The model under review builds one solid part; all positions refer to its coordinate system, in mm. A direction names the side the tool comes from. Give positions to 0.01 mm unless a question says otherwise; leave off trailing zeros. Loops run counter-clockwise (first coordinate to the right, second up) from the corner with the lowest first, then second, coordinate; pieces in that order, holes last. Notation, with made-up numbers: (22, -13) - (50, -13) arc R20 ccw to (50, 10) - close; hole circle Ø7 at (-34, -38). An arc over 180 degrees is marked (long way). Return JSON: item names as keys, results as strings. Group by question number.
from build123d import *

# Parameters (mm, degrees)
SKETCH1_W             = 60
SKETCH1_H             = 50
BOSS_EXTRUDE1_DEPTH   = 3
SKETCH2_W             = 10
SKETCH2_H             = 3
CUT_EXTRUDE1_DEPTH    = 3
CAVITY3_START         = -30
CAVITY3_OUTLINE_W     = 7
CAVITY3_OUTLINE_H     = 3
CAVITY3_OUTLINE_W_2   = 10
CAVITY3_DEPTH         = 3
CAVITY3_START_2       = 27
CAVITY3_2_OUTLINE_W   = 7
CAVITY3_2_OUTLINE_H   = 3
CAVITY3_2_OUTLINE_W_2 = 10
CAVITY3_2_DEPTH       = 3


# Read off the part's stored shape, not the designer's step: Cavity3
with BuildPart() as part:
    # Sketch1 → Boss-Extrude1 (new body)
    with BuildSketch(Plane.XY):
        Rectangle(SKETCH1_W, SKETCH1_H)
    extrude(amount=BOSS_EXTRUDE1_DEPTH)

    # Sketch2 → Cut-Extrude1 (cut)
    with BuildSketch(Plane.XY.offset(3)):
        with Locations((-15, 23.5)):
            Rectangle(SKETCH2_W, SKETCH2_H)
        with Locations((15, 23.5)):
            Rectangle(SKETCH2_W, SKETCH2_H)
    extrude(amount=-CUT_EXTRUDE1_DEPTH, mode=Mode.SUBTRACT)

    # Cavity3 outline → Cavity3 (cut)
    with BuildSketch(Plane.YZ.offset(CAVITY3_START)):
        with Locations((18.5, 1.5)):
            Rectangle(CAVITY3_OUTLINE_W, CAVITY3_OUTLINE_H)
        with Locations((0, 1.5)):
            Rectangle(CAVITY3_OUTLINE_W_2, CAVITY3_OUTLINE_H)
        with Locations((-20, 1.5)):
            Rectangle(CAVITY3_OUTLINE_W_2, CAVITY3_OUTLINE_H)
    extrude(amount=CAVITY3_DEPTH, mode=Mode.SUBTRACT)

    # Cavity3 2 outline → Cavity3 2 (cut)
    with BuildSketch(Plane.YZ.offset(CAVITY3_START_2)):
        with Locations((18.5, 1.5)):
            Rectangle(CAVITY3_2_OUTLINE_W, CAVITY3_2_OUTLINE_H)
        with Locations((0, 1.5)):
            Rectangle(CAVITY3_2_OUTLINE_W_2, CAVITY3_2_OUTLINE_H)
        with Locations((-20, 1.5)):
            Rectangle(CAVITY3_2_OUTLINE_W_2, CAVITY3_2_OUTLINE_H)
    extrude(amount=CAVITY3_2_DEPTH, mode=Mode.SUBTRACT)


solid = part.part
Item 1: For P1, Ø1.5, axis at y = 17.5, z = 1.5, coming from the +X side; P2, Ø0.9, axis at x = 29, z = 1, coming from the -Y side, all flat-tipped, find the tip position at first contact; note any pin that passes through.
Item 2: For L1, parallel to Y at x = 18.5, z = 0.8; L2, parallel to X at y = -17.5, z = 2.3, list the stretches that pass through material, from the lowest coordinate up. Write a range as from..to.
Item 3: Take a section at C-C (y = -1). State the section outline as (x, z) points.
Item 4: Mouldability with a two-part tool opening along Y and no side actions: class faces 4 (the face through (-30, -10, 1)), 5 (the face through (25, 25, 1)), 6 (the face through (28, -5, 1)) as +Y half, -Y half, draft (parallel to the pull), parting line (faces both ways), or undercut.
Item 5: Take a section at B-B (x = 14). State the section outline as (y, z) points, then the cut area to 3 significant figures.
Item 6: Tool access review of faces 1 (the face through (15, 22, 2)), 2 (the face through (-27, 18, 2)), 3 (the face through (-27, -20, 2)): name each direction out of +Z, -Z, +X, -X, +Y, -Y from which nothing blocks a thin tool from reaching the whole face with its end or side.
Check sheet entries:
{
 "1": {"P1": "stops at x = 27", "P2": "stops at y = -15"},
 "2": {"L1": "y = -25..22", "L2": "x = -27..27"},
 "3": {"outline": "(-27, 0) - (27, 0) - (27, 3) - (-27, 3) - close"},
 "4": {"face 4": "draft", "face 5": "+Y half", "face 6": "undercut"},
 "5": {"outline": "(-25, 0) - (22, 0) - (22, 3) - (-25, 3) - close", "area": "141 mm^2"},
 "6": {"face 1": "+Z, -Z, +Y", "face 2": "+Z, -Z, -X", "face 3": "+Z, -Z, -X, -Y"}
}
